```python
from build123d import *

# Parameters (mm, degrees)
F1_DEPTH    = 1.27
F2_W        = 50.2304956317
F2_H        = 5.3818384185
F3_DEPTH    = 12.7
F5_SIZE     = 2.54
F6_T1_DEPTH = 22.86
F6_T3_DEPTH = 10.6423506607
F6_T5_DEPTH = 18.0818384185


# Not quite as in the source:
# - a fillet or chamfer that OpenCascade refuses, or shapes differently, is made with other operations: its cross-section is extruded or revolved along the edge and cut away or added


with BuildPart() as f1:
    # F0 (on Front) → F1 (new body)
    with BuildSketch(Plane.XZ):
        with BuildLine():
            ThreePointArc((3.2290674407, 2.4202670825), (3.8285241608, 1.2755281407), (4.0354143885, 0))
            ThreePointArc((4.0354143885, 0), (3.8285241608, -1.2755281407), (3.2290674407, -2.4202670825))
            Line((3.2290674407, -2.4202670825), (3.2290674407, -2.6700689923))
            Line((3.2290674407, -2.6700689923), (53.7696667016, -2.6700689923))
            Line((53.7696667016, -2.6700689923), (53.7696667016, 2.4202670825))
            Line((53.7696667016, 2.4202670825), (3.2290674407, 2.4202670825))
        make_face()
    extrude(amount=F1_DEPTH)


with BuildPart() as f3:
    # F2 (on face) → F3 (new body)
    with BuildSketch(Plane.XZ.offset(1.27)):
        with Locations((-25.1152478158, 2.6909192093)):
            Rectangle(F2_W, F2_H)
    extrude(amount=F3_DEPTH)

    # F5
    f5_edges = [f3.edges().sort_by_distance(p)[0] for p in [
        (-25.115248, -1.27, 0),
        (0, -1.27, 2.690919),
        (-25.115248, -1.27, 5.381838),
        (-50.230496, -1.27, 2.690919),
    ]]
    chamfer(f5_edges, length=F5_SIZE)

    # F6: fillet of radius 2.54 on 4 edges, made by hand

    # F6_s2 → F6_t1 (cut)
    with BuildSketch(Plane.XZ.offset(-2.54)):
        with BuildLine():
            ThreePointArc((-2.54, 0), (-0.7439487758, 0.7439487758), (0, 2.54))
            Line((0, 2.54), (0, 0))
            Line((0, 0), (-2.54, 0))
        make_face()
        with BuildLine():
            ThreePointArc((0, 2.8418384185), (-0.7439487758, 4.6378896428), (-2.54, 5.3818384185))
            Line((-2.54, 5.3818384185), (0, 5.3818384185))
            Line((0, 5.3818384185), (0, 2.8418384185))
        make_face()
    extrude(amount=F6_T1_DEPTH, mode=Mode.SUBTRACT)

    # F6_s4 → F6_t3 (cut)
    with BuildSketch(Plane.XY.offset(-2.6302561211)):
        with BuildLine():
            ThreePointArc((0, -4.8621024484), (-0.1933459874, -3.8900865302), (-0.7439487758, -3.0660512242))
            Line((-0.7439487758, -3.0660512242), (0, -3.81))
            Line((0, -3.81), (0, -4.8621024484))
        make_face()
    extrude(amount=F6_T3_DEPTH, mode=Mode.SUBTRACT)

    # F6_s6 → F6_t5 (cut)
    with BuildSketch(Plane.XY.offset(-6.35)):
        with BuildLine():
            ThreePointArc((-2.54, -13.97), (-0.7439487758, -13.2260512242), (0, -11.43))
            Line((0, -11.43), (0, -13.97))
            Line((0, -13.97), (-2.54, -13.97))
        make_face()
    extrude(amount=F6_T5_DEPTH, mode=Mode.SUBTRACT)


solid = f3.part
```
Build history of the part. All positions in model axes, mm. Give positions to 0.01 mm unless a question says otherwise; leave off trailing zeros. Loops run counter-clockwise (first coordinate to the right, second up) from the corner with the lowest first, then second, coordinate; pieces in that order, holes last.
1) Band-saw the part on A-A on x = -15. List the corners of the cut face in (y, z), then the cut area to 3 significant figures.
Values follow:
outline: (-13.97, 0) - (-3.81, 0) - (-1.27, 2.54) - (-1.27, 2.84) - (-3.81, 5.38) - (-13.97, 5.38) - close
area: 61.9 mm2
2) Probe line 1 along X through (y, z) = (-9.25, 2.45); line 2 along Y through (x, z) = (-27.5, 2.85); line 3 along X through (y, z) = (-3.5, 0.7). List the from-to ranges inside material, lowest first.
Values follow:
line 1: x = -50.23 to 0
line 2: y = -13.97 to -1.28
line 3: x = -49.92 to -0.79
3) Two-plate mould, pull along Z, no slides. Class faces 1 (the face through (-49.22, -2.8, 2.65)), 2 (the face through (-27, -9, 0)), 3 (the face through (-0.724, -8.442, 4.618)): released by +Z, released by -Z, zero draft, split by the parting line, or undercut.
Values follow:
face 1: zero draft
face 2: released by -Z
face 3: released by +Z
4) Band-saw the part on C-C on y = -2.25. List the corners of the cut face in (x, z), then the cut area to 3 significant figures.
Values follow:
outline: (-48.67, 1.56) - (-1.56, 1.56) - (-1.56, 3.82) - (-48.67, 3.82) - close
area: 107 mm2
5) Drop flat-ended pins along their axis: P1, Ø3, axis at y = -3, z = 3, coming from the +X side; P2, Ø2, axis at x = -40, z = 1.5, coming from the +Y side. Give the stop position or say it passes through.
Values follow:
P1: stops at x = -0.03
P2: stops at y = -1.31
6) Band-saw the part on B-B on z = 4.15. List the corners of the cut face in (x, y).
Values follow:
outline: (-50.23, -13.97) - (-2.54, -13.97) arc R2.54 ccw to (-0.36, -12.74) - (-0.36, -3.55) arc R2.54 ccw to (-0.74, -3.07) - (-1.23, -2.58) - (-49, -2.58) - (-50.23, -3.81) - close
